```python
from build123d import *

# Parameters (mm, degrees)
SKETCH_1_W          = 30
SKETCH_1_H          = 28
EXTRUDE_1_DEPTH     = 10
CUT_EXTRUDE_2_DEPTH = 0.8
M1_4X0_3_2_D        = 1.1
M1_4X0_3_2_DEPTH    = 3.7
M1_4X0_3_2_TIP      = 0.33047334
CUT_EXTRUDE_3_DEPTH = 4
CUT_EXTRUDE_4_DEPTH = 0.5
SKETCH_12_W         = 30
SKETCH_12_H         = 4.25
CUT_EXTRUDE_5_DEPTH = 10
SKETCH_13_R         = 1.7
CUT_EXTRUDE_6_DEPTH = 10
SKETCH_14_W         = 23
SKETCH_14_H         = 23.75
CUT_EXTRUDE_7_DEPTH = 5
CUT_EXTRUDE_9_DEPTH = 3
SKETCH_20_W         = 7
SKETCH_20_H         = 23.75
SKETCH_20_R         = 1.7
EXTRUDE_3_DEPTH     = 4.1
SKETCH_23_W         = 4
SKETCH_23_H         = 23.75
EXTRUDE_4_DEPTH     = 9.1


with BuildPart() as part:
    # 草图1 → 凸台-拉伸1 (new body)
    with BuildSketch(Plane.XY):
        with Locations((7.449728974, 2.736434109)):
            Rectangle(SKETCH_1_W, SKETCH_1_H)
    extrude(amount=EXTRUDE_1_DEPTH)

    # 草图2 → 切除-拉伸2 (cut)
    with BuildSketch(Plane(origin=(0, 0, 0), x_dir=(-1, 0, 0), z_dir=(0, 0, -1))):
        with BuildLine():
            Line((5.050271026, 16.736434109), (-15.449728974, 16.736434109))
            Line((-15.449728974, 16.736434109), (-15.449728974, 3.736434109))
            ThreePointArc((-15.449728974, 3.736434109), (-14.571049317, 1.615113765), (-12.449728974, 0.736434109))
            Line((-12.449728974, 0.736434109), (2.050271026, 0.736434109))
            ThreePointArc((2.050271026, 0.736434109), (4.17159137, 1.615113765), (5.050271026, 3.736434109))
            Line((5.050271026, 3.736434109), (5.050271026, 16.736434109))
        make_face()
    extrude(amount=-CUT_EXTRUDE_2_DEPTH, mode=Mode.SUBTRACT)

    # M1.4x0.3 螺纹孔2
    with Locations(Plane(origin=(0, 0, 0.8), x_dir=(-1, 0, 0), z_dir=(0, 0, -1))):
        with Locations((-12.199728974, 8.736434109), (1.800271026, 8.736434109)):
            Hole(M1_4X0_3_2_D / 2, depth=M1_4X0_3_2_DEPTH)
            with Locations((0, 0, -(M1_4X0_3_2_DEPTH + M1_4X0_3_2_TIP / 2))):  # 118° drill point
                Cone(0, M1_4X0_3_2_D / 2, M1_4X0_3_2_TIP, mode=Mode.SUBTRACT)

    # 草图10 → 切除-拉伸3 (cut)
    with BuildSketch(Plane(origin=(0, 16.736434109, 0), x_dir=(1, 0, 0), z_dir=(0, 1, 0))):
        with BuildLine():
            Line((9.249728974, -0.8), (8.149728974, -0.8))
            Line((8.149728974, -0.8), (8.149728974, -3.7))
            ThreePointArc((8.149728974, -3.7), (8.07901805, -3.870710433), (8.249728974, -3.800000693))
            Line((8.249728974, -3.800000693), (9.14947862, -3.800000693))
            ThreePointArc((9.14947862, -3.800000693), (9.320100726, -3.870799843), (9.249728974, -3.700001016))
            Line((9.249728974, -3.700001016), (9.249728974, -0.8))
        make_face()
        with BuildLine():
            Line((1.149728974, -0.8), (2.249728974, -0.8))
            Line((2.249728974, -0.8), (2.249728974, -3.696415438))
            ThreePointArc((2.249728974, -3.696415438), (2.32297432, -3.873245346), (2.146144411, -3.8))
            Line((2.146144411, -3.8), (1.245429293, -3.8))
            ThreePointArc((1.245429293, -3.8), (1.082058629, -3.867670345), (1.149728974, -3.704299681))
            Line((1.149728974, -3.704299681), (1.149728974, -0.8))
        make_face()
    extrude(amount=-CUT_EXTRUDE_3_DEPTH, mode=Mode.SUBTRACT)

    # 草图11 → 切除-拉伸4 (cut)
    with BuildSketch(Plane(origin=(0, 0, 0), x_dir=(-1, 0, 0), z_dir=(0, 0, -1))):
        with BuildLine():
            Line((-7.549728974, -2.063565891), (-2.849728974, -2.063565891))
            ThreePointArc((-2.849728974, -2.063565891), (-2.422952278, -2.240342587), (-2.599728974, -1.813565891))
            Line((-2.599728974, -1.813565891), (-2.599728974, 0.736434109))
            Line((-2.599728974, 0.736434109), (-7.799728974, 0.736434109))
            Line((-7.799728974, 0.736434109), (-7.799728974, -1.813565891))
            ThreePointArc((-7.799728974, -1.813565891), (-7.976505669, -2.240342587), (-7.549728974, -2.063565891))
        make_face()
    extrude(amount=-CUT_EXTRUDE_4_DEPTH, mode=Mode.SUBTRACT)

    # 草图12 → 切除-拉伸5 (cut)
    with BuildSketch(Plane(origin=(0, 0, 0), x_dir=(-1, 0, 0), z_dir=(0, 0, -1))):
        with Locations((-7.449728974, -9.138565891)):
            Rectangle(SKETCH_12_W, SKETCH_12_H)
    extrude(amount=-CUT_EXTRUDE_5_DEPTH, mode=Mode.SUBTRACT)

    # 草图13 → 切除-拉伸6 (cut)
    with BuildSketch(Plane(origin=(0, 0, 0), x_dir=(-1, 0, 0), z_dir=(0, 0, -1))):
        with Locations((-18.199728974, 9.686434109)):
            Circle(SKETCH_13_R)
    extrude(amount=-CUT_EXTRUDE_6_DEPTH, mode=Mode.SUBTRACT)

    # 草图14 → 切除-拉伸7 (cut)
    with BuildSketch(Plane.XY.offset(10)):
        with Locations((3.949728974, 4.861434109)):
            Rectangle(SKETCH_14_W, SKETCH_14_H)
    extrude(amount=-CUT_EXTRUDE_7_DEPTH, mode=Mode.SUBTRACT)

    # 草图16 → 切除-拉伸9 (cut)
    with BuildSketch(Plane.XY.offset(5)):
        with BuildLine():
            Line((-1.300271026, -7.013565891), (11.699728974, -7.013565891))
            Line((11.699728974, -7.013565891), (11.699728974, -0.513565891))
            ThreePointArc((11.699728974, -0.513565891), (5.199728974, 5.986434109), (-1.300271026, -0.513565891))
            Line((-1.300271026, -0.513565891), (-1.300271026, -7.013565891))
        make_face()
    extrude(amount=-CUT_EXTRUDE_9_DEPTH, mode=Mode.SUBTRACT)

    # 草图20 → 凸台-拉伸3 (add)
    with BuildSketch(Plane.XY.offset(10)):
        with Locations((18.949728974, 4.861434109)):
            Rectangle(SKETCH_20_W, SKETCH_20_H)
        with Locations(Location((18.199728974, 9.686434109, 0), (0, 0, 180))):
            Circle(SKETCH_20_R, mode=Mode.SUBTRACT)
    extrude(amount=EXTRUDE_3_DEPTH)

    # 草图23 → 凸台-拉伸4 (add)
    with BuildSketch(Plane.XY.offset(5)):
        with Locations((-5.550271026, 4.861434109)):
            Rectangle(SKETCH_23_W, SKETCH_23_H)
    extrude(amount=EXTRUDE_4_DEPTH)


solid = part.part
```
Work out the finished part from the listing and answer in its coordinate system (mm). A direction names the side the tool comes from. Give positions to 0.01 mm unless a question says otherwise; leave off trailing zeros. Loops run counter-clockwise (first coordinate to the right, second up) from the corner with the lowest first, then second, coordinate; pieces in that order, holes last. Notation, with made-up numbers: (-22, -24.75) -> (-7, -24.75) arc R18 cw to (-7, -5.75) -> close; hole circle Ø5 at (83, 75). An arc over 180 degrees is marked (long way). Put each result on its own line as item: value. Start each with the question number.
Item 1: The part is cut by section A-A (y = 7.5). Give the vertices of the cut face in (x, z).
Item 2: Find the intervals of material crossed by L1, parallel to X at y = 15.5, z = 1.5; L2, parallel to X at y = 2, z = 6; L3, parallel to Z at x = 13.5, y = 8.5, in increasing order. Write a range as [from, to].
Item 3: The part is cut by section B-B (x = -0.75). Give the vertices of the cut face in (y, z).
Item 4: Each of these flat-tipped pins is pushed along its axis until it touches: P1, Ø0.7, axis at x = 9, y = 14, coming from the -Z side; P2, Ø2, axis at x = -1.5, z = 10.5, coming from the +Y side. Where does it stop, or does it pass through?
Item 5: The part is cut by section C-C (y = 0). Give the vertices of the cut face in (x, z).
Item 6: The part is cut by section D-D (x = 3.25). Give the vertices of the cut face in (y, z), then the cut area to 3 significant figures.
Item 7: The mould has two halves that part along X. Classify faces 4 (the face through (-7.55, 5, 7)), 5 (the face through (19, 5, 14.1)), 6 (the face through (11.7, -4, 4)): released by +X, released by -X, zero draft, split by the parting line, or undercut.
Item 8: Which of the six approach directions +Z, -Z, +X, -X, +Y, -Y give full straight-line access (tool end or side, diameter ignored) to faces 1 (the face through (11, 16.736, 4)), 2 (the face through (5, 0, 2)), 3 (the face through (2.25, 15, 2))?
Answers below:
1. outline: (-7.55, 0) -> (-5.05, 0) -> (-5.05, 0.8) -> (15.45, 0.8) -> (15.45, 0) -> (22.45, 0) -> (22.45, 14.1) -> (15.45, 14.1) -> (15.45, 5) -> (-3.55, 5) -> (-3.55, 14.1) -> (-7.55, 14.1) -> close
2. L1: [-7.55, 1.15], [2.25, 8.15], [9.25, 22.45]
2. L2: [-7.55, -3.55], [15.45, 22.45]
2. L3: [0.8, 5]
3. outline: (-7.01, 0) -> (0.74, 0) -> (0.74, 0.8) -> (16.74, 0.8) -> (16.74, 5) -> (2.1, 5) -> (2.1, 2) -> (-7.01, 2) -> close
4. P1: z = 0.8
4. P2: through
5. outline: (-7.55, 0) -> (2.6, 0) -> (2.6, 0.5) -> (7.8, 0.5) -> (7.8, 0) -> (22.45, 0) -> (22.45, 14.1) -> (15.45, 14.1) -> (15.45, 5) -> (11.68, 5) -> (11.68, 2) -> (-1.28, 2) -> (-1.28, 5) -> (-3.55, 5) -> (-3.55, 14.1) -> (-7.55, 14.1) -> close
6. outline: (-7.01, 0) -> (-2.06, 0) -> (-2.06, 0.5) -> (0.74, 0.5) -> (0.74, 0.8) -> (16.74, 0.8) -> (16.74, 5) -> (5.69, 5) -> (5.69, 2) -> (-7.01, 2) -> close
6. area: 66.4 mm2
7. face 4: released by -X
7. face 5: zero draft
7. face 6: undercut
8. face 1: +Z, -Z, +X, -X, +Y
8. face 2: +Z, -Y
8. face 3: -Z, +Y
